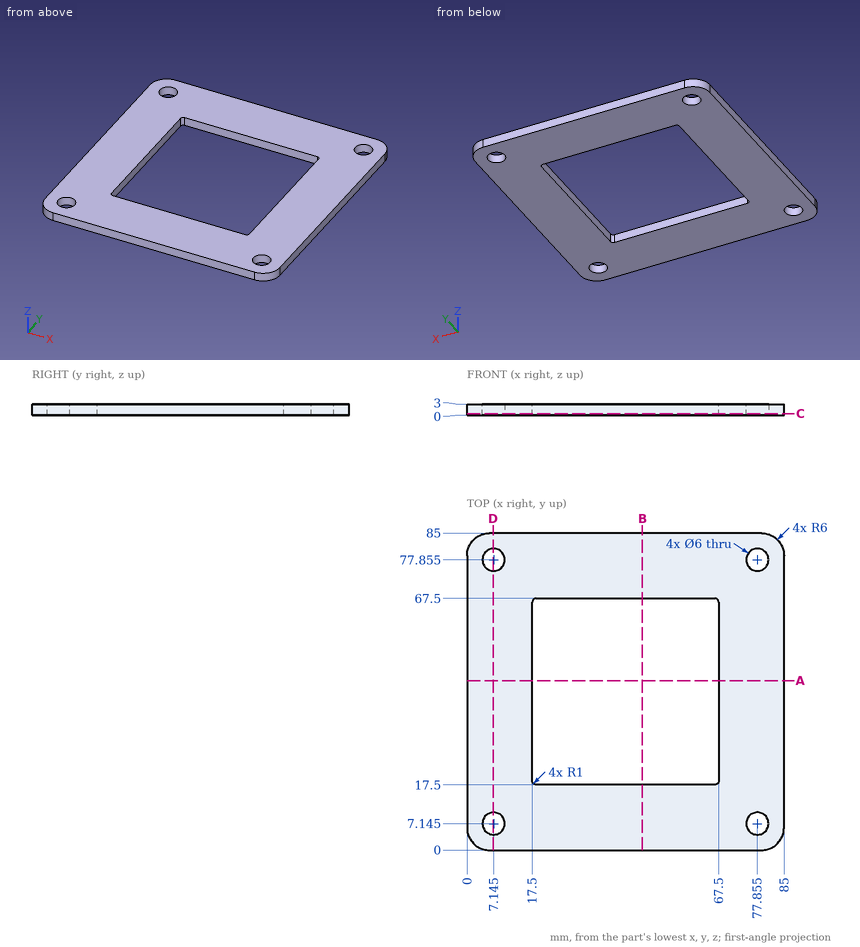
Design review of the part shown in the three views and the two pictorial views. Dimensions are in mm from the part's minimum x, y and z. Round coordinates to 2 decimals unless told otherwise and drop trailing zeros. Order: outer loops, then holes, each group sorted by start corner. A loop starts at its lowest first (then second) coordinate and runs counter-clockwise, first axis right, second up.
(1) Take a section at D-D, the plane x = 7. State the section outline as (y, z) points, plus the area to 3 significant figures.
Working result:
outline: (0, 0) - (4.15, 0) - (4.15, 3) - (0, 3) - close; (10.14, 0) - (74.86, 0) - (74.86, 3) - (10.14, 3) - close; (80.85, 0) - (85, 0) - (85, 3) - (80.85, 3) - close
area: 219 mm2
(2) Take a section at C-C, the plane z = 0.45. State the section outline as (x, y) points (1 decimal), plus the area to 3 significant figures.
Working result:
outline: (0, 6) arc R6 ccw to (6, 0) - (79, 0) arc R6 ccw to (85, 6) - (85, 79) arc R6 ccw to (79, 85) - (6, 85) arc R6 ccw to (0, 79) - close; hole circle Ø6 at (7.1, 7.1); hole circle Ø6 at (7.1, 77.9); hole (17.5, 18.5) arc R1 ccw to (18.5, 17.5) - (66.5, 17.5) arc R1 ccw to (67.5, 18.5) - (67.5, 66.5) arc R1 ccw to (66.5, 67.5) - (18.5, 67.5) arc R1 ccw to (17.5, 66.5) - close; hole circle Ø6 at (77.9, 7.1); hole circle Ø6 at (77.9, 77.9)
area: 4,580 mm2
(3) Take a section at A-A, the plane y = 45.5. State the section outline as (x, z) points.
Working result:
outline: (0, 0) - (17.5, 0) - (17.5, 3) - (0, 3) - close; (67.5, 0) - (85, 0) - (85, 3) - (67.5, 3) - close
(4) Wall thickness on L1, parallel to X at y = 56, z = 1.8; L2, parallel to X at y = 6, z = 1.4: over which ranges is each line inside the solid? List them lowest first.
Working result:
L1: x = 0 to 17.5, 67.5 to 85
L2: x = 0 to 4.37, 9.92 to 75.08, 80.63 to 85
